Build history of the part. All positions in model axes, mm. A direction names the side the tool comes from. Round coordinates to 2 decimals unless told otherwise and drop trailing zeros. Loops run counter-clockwise (first coordinate to the right, second up) from the corner with the lowest first, then second, coordinate; pieces in that order, holes last. Notation, with made-up numbers: (54, 18) -> (88, 18) arc R22 cw to (88, 31) -> close; hole circle Ø8 at (0, -27.5). An arc over 180 degrees is marked (long way). Put each result on its own line as item: value. Start each with the question number.
Item 1: Flat gauge pins, fed straight in: pin 1 Ø10 at (x, z) = (40.5, -10) entering from +Y; pin 2 Ø1.5 at (x, z) = (49, -0.5) entering from +Y; pin 3 Ø6.5 at (x, y) = (56.84, 33.58) entering from -Z; pin 4 Ø4 at (x, y) = (39.34, 26.48) entering from +Z. Where does each tip first touch, or does it go through?
Item 2: Drill centre lines: probe 1 along Z at (x, y) = (56, 25.5); probe 2 along X at (y, z) = (32.5, 2); probe 3 along X at (y, z) = (27, 2). Where is each one in solid material? Low to high. Write a range as [from, to].
Item 3: Cut at B-B, the plane x = 39. List the corners of the cut face in (y, z), plus the area to 3 significant figures.
Item 4: Cut at D-D, the plane z = -7.75. List the corners of the cut face in (x, y), plus the area to 3 significant figures.
Item 5: Cut at C-C, the plane y = 28. List the corners of the cut face in (x, z).
Item 6: Pull direction X, two halves, no side cores. Call faces 6 (the flat face through (47.56, 31.245, 1.972)), 7 (the cylindrical face through (56.269, 23.894, 2.028)), 8 (the flat face through (45, 26, -9.9)): +X half, -X half, draft (parallel to the pull), parting line (faces both ways), or undercut.
Item 7: Cut at A-A, the plane y = 24.5. List the corners of the cut face in (x, z).
Item 8: Tool access for faces 1 (the flat face through (48, 28, 4)), 2 (the cylindrical face through (51.497, 33.22, 2.028)), 3 (the flat face through (49, 23.292, 2)), 4 (the cylindrical face through (45.109, 29.046, -11.379)), 5 (the cylindrical face through (45.45, 28.04, -4.88)): list every direction of +Z, -Z, +X, -X, +Y, -Y with a clear straight run to the whole face (end or side of a thin tool).
```python
from build123d import *

# Parameters (mm, degrees)
SKETCH1_R           = 2.5
BOSS_EXTRUDE1_DEPTH = 4
FILLET1_R           = 2
BOSS_EXTRUDE2_START = -3.9
SKETCH2_R           = 1
BOSS_EXTRUDE2_DEPTH = 10
SKETCH3_R           = 2
BOSS_EXTRUDE3_DEPTH = 3


with BuildPart() as part:
    # Sketch1 → Boss-Extrude1 (new body)
    with BuildSketch(Plane.XY):
        with BuildLine():
            Line((56.839071038, 28.579919803), (56.839071038, 23.292312115))
            Line((56.839071038, 23.292312115), (43.08257304, 23.292312115))
            ThreePointArc((43.08257304, 23.292312115), (34.429928081, 26.628647856), (43.273147001, 29.420937259))
            Line((43.273147001, 29.420937259), (51.8645252, 33.076041142))
            ThreePointArc((51.8645252, 33.076041142), (60.191727201, 37.289326312), (56.839071038, 28.579919803))
        make_face()
        with Locations((39.340592987, 26.475947236)):
            Circle(SKETCH1_R, mode=Mode.SUBTRACT)
        with Locations((56.839071038, 33.579919803)):
            Circle(SKETCH1_R, mode=Mode.SUBTRACT)
    extrude(amount=BOSS_EXTRUDE1_DEPTH)

    # Fillet1
    fillet1_edges = [part.edges().sort_by_distance(p)[0] for p in [
        (56.839071038, 28.579919803, 2),
        (56.839071038, 23.292312115, 2),
        (43.08257304, 23.292312115, 2),
        (43.273147001, 29.420937259, 2),
        (51.8645252, 33.076041142, 2),
    ]]
    fillet(fillet1_edges, radius=FILLET1_R)

    # Sketch2 → Boss-Extrude2 (add)
    with BuildSketch(Plane.XY.offset(4).offset(BOSS_EXTRUDE2_START)):
        with Locations((46.18381054, 27.359606691)):
            Circle(SKETCH2_R)
    extrude(amount=-BOSS_EXTRUDE2_DEPTH)

    # Sketch3 → Boss-Extrude3 (add)
    with BuildSketch(Plane(origin=(0, 0, -9.9), x_dir=(-1, 0, 0), z_dir=(0, 0, -1))):
        with Locations((-46.18381054, 27.359606691)):
            Circle(SKETCH3_R)
    extrude(amount=BOSS_EXTRUDE3_DEPTH)


solid = part.part
```
Reply:
1. pin 1: stops at y = 29.24
1. pin 2: stops at y = 32.1
1. pin 3: stops at z = 0
1. pin 4: passes through
2. probe 1: z = [0, 4]
2. probe 2: x = [50.51, 54.58], [59.09, 61.72]
2. probe 3: x = [34.46, 36.9], [41.79, 56.84]
3. outline: (21.57, 0) -> (24, 0) -> (24, 4) -> (21.57, 4) -> close; (28.95, 0) -> (31.38, 0) -> (31.38, 4) -> (28.95, 4) -> close
3. area: 19.4 mm^2
4. outline: circle Ø2 at (46.18, 27.36)
4. area: 3.14 mm^2
5. outline: (34.67, 0) -> (37.36, 0) -> (37.36, 4) -> (34.67, 4) -> close; (41.32, 0) -> (45.42, 0) -> (45.42, -9.9) -> (44.29, -9.9) -> (44.29, -12.9) -> (48.08, -12.9) -> (48.08, -9.9) -> (46.95, -9.9) -> (46.95, 0) -> (57.19, 0) -> (57.19, 4) -> (41.32, 4) -> close
6. face 6: undercut
6. face 7: +X half
6. face 8: draft
7. outline: (34.84, 0) -> (37.81, 0) -> (37.81, 4) -> (34.84, 4) -> close; (40.87, 0) -> (56.68, 0) -> (56.68, 4) -> (40.87, 4) -> close
8. face 1: +Z, +X, -X, +Y, -Y
8. face 2: +Z, -Z, -X, +Y
8. face 3: +Z, -Z, +X, -Y
8. face 4: -Z
8. face 5: none
